from build123d import *

# Parameters (mm, degrees)
BOSS_EXTRUDE1_DEPTH = 3.175
CUT_EXTRUDE4_DEPTH  = 235.179100055
SKETCH5_R           = 2.54
CUT_EXTRUDE3_DEPTH  = 235.179100055
SKETCH4_R           = 2.159
CUT_EXTRUDE2_DEPTH  = 235.179100055
FILLET1_R           = 25.4


with BuildPart() as part:
    # Sketch1 → Boss-Extrude1 (new body)
    with BuildSketch(Plane(origin=(0, 0, 0), x_dir=(1, 0, 0), z_dir=(0, 1, 0))):
        Polygon((-139.7, 73.520142619), (-121.739487758, 91.480654861), (121.739487758, 91.480654861), (139.7, 73.520142619), (139.7, -169.958832897), (121.739487758, -187.919345139), (-121.739487758, -187.919345139), (-139.7, -169.958832897), align=None)
    extrude(amount=BOSS_EXTRUDE1_DEPTH)

    # Sketch2 → Cut-Extrude4 (cut, through all)
    with BuildSketch(Plane(origin=(0, 3.175, 0), x_dir=(1, 0, 0), z_dir=(0, 1, 0))):
        Polygon((-103.778975516, 37.599118134), (-114.3, 27.07809365), (-114.3, -123.516783928), (-103.778975516, -134.037808413), (-85.818463274, -151.998320655), (-75.297438789, -162.519345139), (75.297438789, -162.519345139), (85.818463274, -151.998320655), (103.778975516, -134.037808413), (114.3, -123.516783928), (114.3, 27.07809365), (103.778975516, 37.599118134), (85.818463274, 55.559630377), (75.297438789, 66.080654861), (-75.297438789, 66.080654861), (-85.818463274, 55.559630377), align=None)
    extrude(amount=-CUT_EXTRUDE4_DEPTH, mode=Mode.SUBTRACT)

    # Sketch5 → Cut-Extrude3 (cut, through all)
    with BuildSketch(Plane(origin=(0, 3.175, 0), x_dir=(1, 0, 0), z_dir=(0, 1, 0))):
        with Locations(Location((-121.739487758, 73.520142619, 0), (0, 0, 270))):
            Circle(SKETCH5_R)
        with Locations(Location((-103.778975516, 55.559630377, 0), (0, 0, 270))):
            Circle(SKETCH5_R)
        with Locations(Location((103.778975516, 55.559630377, 0), (0, 0, 90))):
            Circle(SKETCH5_R)
        with Locations(Location((121.739487758, 73.520142619, 0), (0, 0, 90))):
            Circle(SKETCH5_R)
        with Locations(Location((121.739487758, -169.958832897, 0), (0, 0, 270))):
            Circle(SKETCH5_R)
        with Locations(Location((103.778975516, -151.998320655, 0), (0, 0, 270))):
            Circle(SKETCH5_R)
        with Locations(Location((-103.778975516, -151.998320655, 0), (0, 0, 90))):
            Circle(SKETCH5_R)
        with Locations(Location((-121.739487758, -169.958832897, 0), (0, 0, 90))):
            Circle(SKETCH5_R)
    extrude(amount=-CUT_EXTRUDE3_DEPTH, mode=Mode.SUBTRACT)

    # Sketch4 → Cut-Extrude2 (cut, through all)
    with BuildSketch(Plane(origin=(0, 3.175, 0), x_dir=(1, 0, 0), z_dir=(0, 1, 0))):
        with Locations(Location((0, 81.320654861, 0), (0, 0, 270))):
            Circle(SKETCH4_R)
        with Locations(Location((-44.45, 81.320654861, 0), (0, 0, 270))):
            Circle(SKETCH4_R)
        with Locations(Location((44.45, 81.320654861, 0), (0, 0, 270))):
            Circle(SKETCH4_R)
        with Locations(Location((-22.225, 81.320654861, 0), (0, 0, 270))):
            Circle(SKETCH4_R)
        with Locations(Location((22.225, 81.320654861, 0), (0, 0, 270))):
            Circle(SKETCH4_R)
        with Locations(Location((-129.54, -48.219345139, 0), (0, 0, 270))):
            Circle(SKETCH4_R)
        with Locations(Location((-129.54, -25.994345139, 0), (0, 0, 270))):
            Circle(SKETCH4_R)
        with Locations(Location((-129.54, -3.769345139, 0), (0, 0, 270))):
            Circle(SKETCH4_R)
        with Locations(Location((129.54, -48.219345139, 0), (0, 0, 270))):
            Circle(SKETCH4_R)
        with Locations(Location((129.54, -25.994345139, 0), (0, 0, 270))):
            Circle(SKETCH4_R)
        with Locations(Location((129.54, -3.769345139, 0), (0, 0, 270))):
            Circle(SKETCH4_R)
        with Locations(Location((129.54, -92.669345139, 0), (0, 0, 90))):
            Circle(SKETCH4_R)
        with Locations(Location((129.54, -70.444345139, 0), (0, 0, 90))):
            Circle(SKETCH4_R)
        with Locations(Location((-129.54, -92.669345139, 0), (0, 0, 90))):
            Circle(SKETCH4_R)
        with Locations(Location((-129.54, -70.444345139, 0), (0, 0, 90))):
            Circle(SKETCH4_R)
        with Locations(Location((22.225, -177.759345139, 0), (0, 0, 90))):
            Circle(SKETCH4_R)
        with Locations(Location((-22.225, -177.759345139, 0), (0, 0, 90))):
            Circle(SKETCH4_R)
        with Locations(Location((44.45, -177.759345139, 0), (0, 0, 90))):
            Circle(SKETCH4_R)
        with Locations(Location((-44.45, -177.759345139, 0), (0, 0, 90))):
            Circle(SKETCH4_R)
        with Locations(Location((0, -177.759345139, 0), (0, 0, 90))):
            Circle(SKETCH4_R)
        with Locations(Location((-66.675, 81.320654861, 0), (0, 0, 270))):
            Circle(SKETCH4_R)
        with Locations(Location((66.675, 81.320654861, 0), (0, 0, 270))):
            Circle(SKETCH4_R)
        with Locations(Location((-129.54, 18.455654861, 0), (0, 0, 270))):
            Circle(SKETCH4_R)
        with Locations(Location((129.54, 18.455654861, 0), (0, 0, 270))):
            Circle(SKETCH4_R)
        with Locations(Location((129.54, -114.894345139, 0), (0, 0, 90))):
            Circle(SKETCH4_R)
        with Locations(Location((66.675, -177.759345139, 0), (0, 0, 90))):
            Circle(SKETCH4_R)
        with Locations(Location((-66.675, -177.759345139, 0), (0, 0, 90))):
            Circle(SKETCH4_R)
        with Locations(Location((-129.54, -114.894345139, 0), (0, 0, 90))):
            Circle(SKETCH4_R)
        with Locations(Location((-129.54, -137.119345139, 0), (0, 0, 270))):
            Circle(SKETCH4_R)
        with Locations(Location((-129.54, 40.680654861, 0), (0, 0, 90))):
            Circle(SKETCH4_R)
        with Locations(Location((129.54, 40.680654861, 0), (0, 0, 270))):
            Circle(SKETCH4_R)
        with Locations(Location((129.54, -137.119345139, 0), (0, 0, 90))):
            Circle(SKETCH4_R)
    extrude(amount=-CUT_EXTRUDE2_DEPTH, mode=Mode.SUBTRACT)

    # Fillet1
    fillet1_edges = [part.edges().sort_by_distance(p)[0] for p in [
        (-75.297438789, 1.5875, -66.080654861),
        (75.297438789, 1.5875, -66.080654861),
        (114.3, 1.5875, -27.07809365),
        (114.3, 1.5875, 123.516783928),
        (75.297438789, 1.5875, 162.519345139),
        (-75.297438789, 1.5875, 162.519345139),
        (-114.3, 1.5875, 123.516783928),
        (-114.3, 1.5875, -27.07809365),
    ]]
    fillet(fillet1_edges, radius=FILLET1_R)


solid = part.part
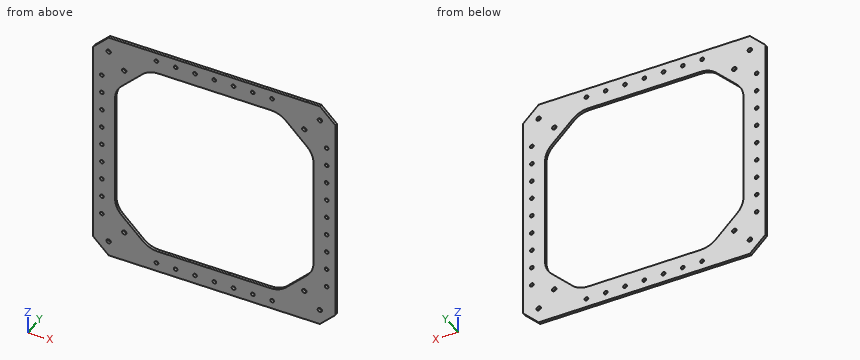
Source: CAD feature listing. Evaluate the final solid. Frame: model axes, mm. Give positions to 0.01 mm unless a question says otherwise; leave off trailing zeros. Loops run counter-clockwise (first coordinate to the right, second up) from the corner with the lowest first, then second, coordinate; pieces in that order, holes last. Notation, with made-up numbers: (38, -8.75) -> (50, -8.75) arc R21 cw to (50, 27.25) -> close; hole circle Ø6 at (-19, -26). An arc over 180 degrees is marked (long way). Use a Markdown table: item, result. Add a question column.
1) Line query: line 1 along X through (y, z) = (1.5, 152); line 2 along X through (y, z) = (2, -12); line 3 along Z through (x, y) = (14.5, 1.4). Output: solid intervals per line, ascending. Write a range as [from, to].
2) Section query A-A, the plane z = -12.5. Return the cut outline in (x, y) (3 decimals), then the cut area to 3 significant figures.
3) Section query C-C, the plane y = 1.9. Count the separate pieces of the cut face and the enclosed holes in it, then the cut area to 3 significant figures.
4) Section query B-B, the plane x = -32.5. Return the cut outline in (y, z) (3 decimals).
Numbers:
| question | item | result |
|---|---|---|
| 1 | line 1 | x = [-139.7, -106.32], [-101.24, -85.82], [85.82, 101.24], [106.32, 139.7] |
| 1 | line 2 | x = [-139.7, -114.3], [114.3, 139.7] |
| 1 | line 3 | z = [-91.48, -66.08], [162.52, 187.92] |
| 2 | outline | (-139.7, 0) -> (-114.3, 0) -> (-114.3, 3.175) -> (-139.7, 3.175) -> close; (114.3, 0) -> (139.7, 0) -> (139.7, 3.175) -> (114.3, 3.175) -> close |
| 2 | area | 161 mm2 |
| 3 | separate pieces | 1 |
| 3 | enclosed holes | 41 |
| 3 | area | 27,700 mm2 |
| 4 | outline | (0, -91.481) -> (3.175, -91.481) -> (3.175, -66.081) -> (0, -66.081) -> close; (0, 162.519) -> (3.175, 162.519) -> (3.175, 187.919) -> (0, 187.919) -> close |
